The figure shows three views and two pictorial views of one solid part (mm, origin at its lowest corner). Answer the questions. A direction names the side the tool comes from. Round coordinates to 2 decimals unless told otherwise and drop trailing zeros. Write each loop counter-clockwise with the first axis right and the second up, starting at its lowest first coordinate (ties: lowest second). Pieces come first, ordered by that corner, then holes.
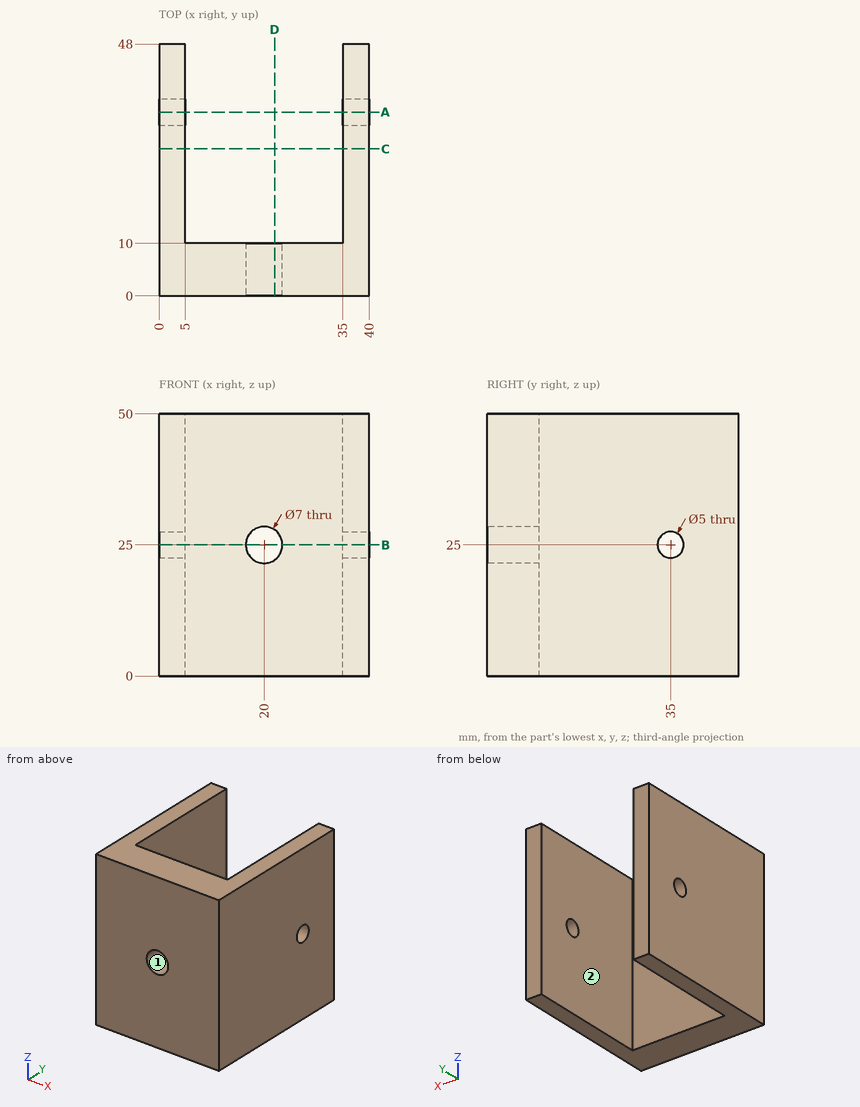
Q1. Section C-C (y = 28) is taken. Determine the outline of the cut face in (x, z), then the cut area to 3 significant figures.
Verdict:
outline: (0, 0) - (5, 0) - (5, 50) - (0, 50) - close; (35, 0) - (40, 0) - (40, 50) - (35, 50) - close
area: 500 mm2
Q2. Which of the six approach directions +Z, -Z, +X, -X, +Y, -Y give full straight-line access (tool end or side, diameter ignored) to the marked faces 1 and 2?
Verdict:
face 1: +Y, -Y
face 2: +Z, -Z, +Y
Q3. Section B-B (z = 25) is taken. Determine the outline of the cut face in (x, y), then the cut area to 3 significant figures.
Verdict:
outline: (0, 0) - (16.5, 0) - (16.5, 10) - (5, 10) - (5, 32.5) - (0, 32.5) - close; (0, 37.5) - (5, 37.5) - (5, 48) - (0, 48) - close; (23.5, 0) - (40, 0) - (40, 32.5) - (35, 32.5) - (35, 10) - (23.5, 10) - close; (35, 37.5) - (40, 37.5) - (40, 48) - (35, 48) - close
area: 660 mm2
Q4. Flat-ended cylindrical pins translate along their axes: pin 1 Ø15 at (x, z) = (19, 17.5) entering from +Y; pin 2 Ø8 at (y, z) = (35, 25) entering from -X. Find the tip coordinate at first contact, or state that the pin passes through.
Verdict:
pin 1: stops at y = 10
pin 2: stops at x = 0
Q5. Section A-A (y = 35) is taken. Determine the outline of the cut face in (x, z), then the cut area to 3 significant figures.
Verdict:
outline: (0, 0) - (5, 0) - (5, 22.5) - (0, 22.5) - close; (0, 27.5) - (5, 27.5) - (5, 50) - (0, 50) - close; (35, 0) - (40, 0) - (40, 22.5) - (35, 22.5) - close; (35, 27.5) - (40, 27.5) - (40, 50) - (35, 50) - close
area: 450 mm2
Q6. Straight lines are drawn through the part: probe 1 along Z at (x, y) = (37.1, 35); probe 2 along X at (y, z) = (18, 23); probe 3 along Z at (x, y) = (20, 4). For each, find the intervals that lie inside material, in ascending order.
Verdict:
probe 1: z = 0 to 22.5, 27.5 to 50
probe 2: x = 0 to 5, 35 to 40
probe 3: z = 0 to 21.5, 28.5 to 50
Q7. Section D-D (x = 22) is taken. Determine the outline of the cut face in (y, z).
Verdict:
outline: (0, 0) - (10, 0) - (10, 22.13) - (0, 22.13) - close; (0, 27.87) - (10, 27.87) - (10, 50) - (0, 50) - close
